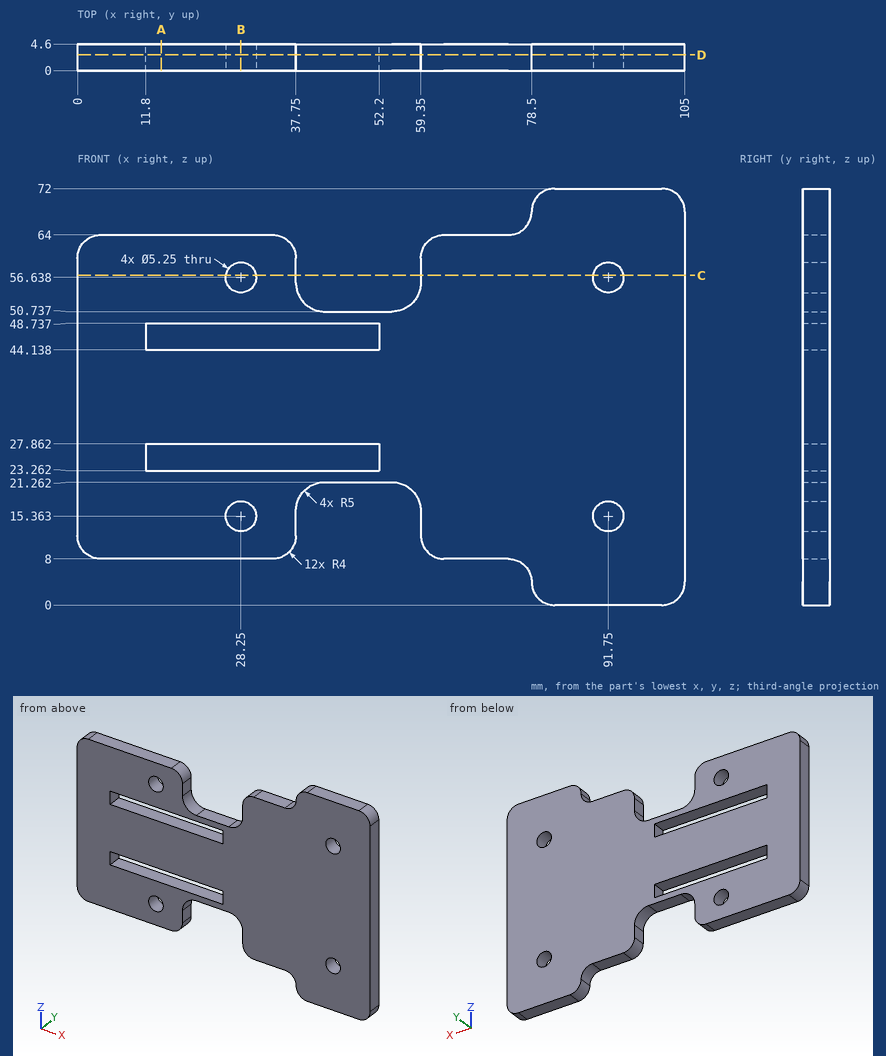
Geometry check sheet. Reference: drawing and pictorial views, mm from the part's lowest x, y, z. Round coordinates to 2 decimals unless told otherwise and drop trailing zeros. Write each loop counter-clockwise with the first axis right and the second up, starting at its lowest first coordinate (ties: lowest second). Pieces come first, ordered by that corner, then holes. Notation, with made-up numbers: (-4, -24.5) -> (32, -24.5) arc R9 ccw to (32, -9.5) -> close; hole circle Ø7 at (26.25, 15.25). An arc over 180 degrees is marked (long way). One line per question, with ' | ' between items. Start each with the question number.
1. Sectioned sample at D-D, the plane y = 2.7. Count the separate pieces of the cut face and the enclosed holes in it, then the cut area to 3 significant figures.
2. Depth check by flat-ended pin: pin 1 (1.5 mm diameter, centred on x = 81.5, y = 4, fed in from -Z); pin 2 (2.5 mm diameter, centred on x = 71, y = 2, fed in from -Z). Enter the tip coordinate at first touch or a pass-through.
3. Sectioned sample at B-B, the plane x = 28.25. Record the cut outline in (y, z).
4. Sectioned sample at A-A, the plane x = 14.5. Record the cut outline in (y, z), then the cut area to 3 significant figures.
5. Sectioned sample at C-C, the plane z = 57. Record the cut outline in (x, y), then the cut area to 3 significant figures.
6. Scan lines: line 1 along Z through (x, y) = (91.75, 1.2); line 2 along Z through (x, y) = (16, 1.55); line 3 along X through (y, z) = (2.6, 27.5). Record each from-to range of solid material in increasing order. Write a range as from..to.
Taken from the geometry:
1) separate pieces: 1 | enclosed holes: 6 | area: 5,270 mm^2
2) pin 1: stops at z = 0.01 | pin 2: stops at z = 8
3) outline: (0, 8) -> (4.6, 8) -> (4.6, 12.74) -> (0, 12.74) -> close; (0, 17.99) -> (4.6, 17.99) -> (4.6, 23.26) -> (0, 23.26) -> close; (0, 27.86) -> (4.6, 27.86) -> (4.6, 44.14) -> (0, 44.14) -> close; (0, 48.74) -> (4.6, 48.74) -> (4.6, 54.01) -> (0, 54.01) -> close; (0, 59.26) -> (4.6, 59.26) -> (4.6, 64) -> (0, 64) -> close
4) outline: (0, 8) -> (4.6, 8) -> (4.6, 23.26) -> (0, 23.26) -> close; (0, 27.86) -> (4.6, 27.86) -> (4.6, 44.14) -> (0, 44.14) -> close; (0, 48.74) -> (4.6, 48.74) -> (4.6, 64) -> (0, 64) -> close | area: 215 mm^2
5) outline: (0, 0) -> (25.65, 0) -> (25.65, 4.6) -> (0, 4.6) -> close; (30.85, 0) -> (37.75, 0) -> (37.75, 4.6) -> (30.85, 4.6) -> close; (59.35, 0) -> (89.15, 0) -> (89.15, 4.6) -> (59.35, 4.6) -> close; (94.35, 0) -> (105, 0) -> (105, 4.6) -> (94.35, 4.6) -> close | area: 336 mm^2
6) line 1: z = 0..12.74, 17.99..54.01, 59.26..72 | line 2: z = 8..23.26, 27.86..44.14, 48.74..64 | line 3: x = 0..11.8, 52.2..105
